from build123d import *

# Parameters (mm, degrees)
BASEFLANGE_W                   = 70
BASEFLANGE_H                   = 531
BASE_FLANGE1_DEPTH             = 2
EDGE_FLANGE1_STRIP_W           = 10
EDGE_FLANGE1_STRIP_H           = 2
EDGE_FLANGE1_STRIP_CUT_DEPTH   = 531
EDGE_FLANGE1_STRIP_2_W         = 10
EDGE_FLANGE1_STRIP_2_H         = 2
EDGE_FLANGE1_STRIP_CUT_2_DEPTH = 531
EDGE_FLANGE1_DEPTH             = 531
EDGE_FLANGE1_BEND_DEPTH        = 531
EDGE_FLANGE2_STRIP_W           = 10
EDGE_FLANGE2_STRIP_H           = 2
EDGE_FLANGE2_STRIP_CUT_DEPTH   = 531
EDGE_FLANGE2_STRIP_2_W         = 10
EDGE_FLANGE2_STRIP_2_H         = 2
EDGE_FLANGE2_STRIP_CUT_2_DEPTH = 531
EDGE_FLANGE2_DEPTH             = 531
EDGE_FLANGE2_BEND_DEPTH        = 531


# Sheet-metal steps are written as plain solids
with BuildPart() as part:
    # BaseFlange → Base-Flange1 (new body)
    with BuildSketch(Plane(origin=(0, 0, 0), x_dir=(1, 0, 0), z_dir=(0, 1, 0))):
        with Locations((0, -265.5)):
            Rectangle(BASEFLANGE_W, BASEFLANGE_H)
    extrude(amount=-BASE_FLANGE1_DEPTH)

    # Edge-Flange1 strip (across the edge) → Edge-Flange1 strip cut (cut)
    with BuildSketch(Plane(origin=(-35, -2, 531), x_dir=(1, 0, 0), z_dir=(0, 0, -1))):
        with Locations((-2, -1)):
            Rectangle(EDGE_FLANGE1_STRIP_W, EDGE_FLANGE1_STRIP_H)
    extrude(amount=EDGE_FLANGE1_STRIP_CUT_DEPTH, mode=Mode.SUBTRACT)

    # Edge-Flange1 strip 2 (across the edge) → Edge-Flange1 strip cut 2 (cut)
    with BuildSketch(Plane(origin=(35, -2, 0), x_dir=(-1, 0, 0), z_dir=(0, 0, 1))):
        with Locations((-2, -1)):
            Rectangle(EDGE_FLANGE1_STRIP_2_W, EDGE_FLANGE1_STRIP_2_H)
    extrude(amount=EDGE_FLANGE1_STRIP_CUT_2_DEPTH, mode=Mode.SUBTRACT)

    # Edge-Flange1 section (across the edge) → Edge-Flange1 (add)
    with BuildSketch(Plane(origin=(-35, -2, 531), x_dir=(1, 0, 0), z_dir=(0, 0, -1))):
        with BuildLine():
            Line((0, 1), (0, 46))
            Line((0, 46), (2, 46))
            Line((2, 46), (2, 1))
            ThreePointArc((2, 1), (2.292893219, 0.292893219), (3, 0))
            Line((3, 0), (3, -2))
            ThreePointArc((3, -2), (0.878679656, -1.121320344), (0, 1))
        make_face()
    extrude(amount=EDGE_FLANGE1_DEPTH)

    # Edge-Flange1 section 2 (across the edge) → Edge-Flange1 bend (add)
    with BuildSketch(Plane(origin=(35, -2, 0), x_dir=(-1, 0, 0), z_dir=(0, 0, 1))):
        with BuildLine():
            Line((0, 1), (0, 46))
            Line((0, 46), (2, 46))
            Line((2, 46), (2, 1))
            ThreePointArc((2, 1), (2.292893219, 0.292893219), (3, 0))
            Line((3, 0), (3, -2))
            ThreePointArc((3, -2), (0.878679656, -1.121320344), (0, 1))
        make_face()
    extrude(amount=EDGE_FLANGE1_BEND_DEPTH)

    # Edge-Flange2 strip (across the edge) → Edge-Flange2 strip cut (cut)
    with BuildSketch(Plane(origin=(-33, -48, 531), x_dir=(0, 1, 0), z_dir=(0, 0, -1))):
        with Locations((-2, -1)):
            Rectangle(EDGE_FLANGE2_STRIP_W, EDGE_FLANGE2_STRIP_H)
    extrude(amount=EDGE_FLANGE2_STRIP_CUT_DEPTH, mode=Mode.SUBTRACT)

    # Edge-Flange2 strip 2 (across the edge) → Edge-Flange2 strip cut 2 (cut)
    with BuildSketch(Plane(origin=(33, -48, 0), x_dir=(0, 1, 0), z_dir=(0, 0, 1))):
        with Locations((-2, -1)):
            Rectangle(EDGE_FLANGE2_STRIP_2_W, EDGE_FLANGE2_STRIP_2_H)
    extrude(amount=EDGE_FLANGE2_STRIP_CUT_2_DEPTH, mode=Mode.SUBTRACT)

    # Edge-Flange2 section (across the edge) → Edge-Flange2 (add)
    with BuildSketch(Plane(origin=(-33, -48, 531), x_dir=(0, 1, 0), z_dir=(0, 0, -1))):
        with BuildLine():
            Line((0, 1), (0, 8))
            Line((0, 8), (2, 8))
            Line((2, 8), (2, 1))
            ThreePointArc((2, 1), (2.292893219, 0.292893219), (3, 0))
            Line((3, 0), (3, -2))
            ThreePointArc((3, -2), (0.878679656, -1.121320344), (0, 1))
        make_face()
    extrude(amount=EDGE_FLANGE2_DEPTH)

    # Edge-Flange2 section 2 (across the edge) → Edge-Flange2 bend (add)
    with BuildSketch(Plane(origin=(33, -48, 0), x_dir=(0, 1, 0), z_dir=(0, 0, 1))):
        with BuildLine():
            Line((0, 1), (0, 8))
            Line((0, 8), (2, 8))
            Line((2, 8), (2, 1))
            ThreePointArc((2, 1), (2.292893219, 0.292893219), (3, 0))
            Line((3, 0), (3, -2))
            ThreePointArc((3, -2), (0.878679656, -1.121320344), (0, 1))
        make_face()
    extrude(amount=EDGE_FLANGE2_BEND_DEPTH)


solid = part.part
Part model, mm, in its own coordinate system. A direction names the side the tool comes from. Coordinates: 2 decimals unless noted, no trailing zeros. Order: outer loops, then holes, each group sorted by start corner. A loop starts at its lowest first (then second) coordinate and runs counter-clockwise, first axis right, second up.
(1) Pull direction X, two halves, no side cores. Call faces 3 (the face through (0, -1, 531)), 4 (the face through (-35, -24, 269)), 5 (the face through (33, -24, 262)): pulls with the +X half, pulls with the -X half, needs draft (parallel to the pull), parting line crosses it, or undercut.
Check sheet entries:
face 3: needs draft
face 4: pulls with the -X half
face 5: undercut
(2) Tool access for faces 1 (the face through (-33, -24, 269)), 2 (the face through (0, -1, 0)): list every direction of +Z, -Z, +X, -X, +Y, -Y with a clear straight run to the whole face (end or side of a thin tool).
Check sheet entries:
face 1: +Z, -Z
face 2: -Z, +X, -X, +Y, -Y
(3) Probe L1, parallel to X at y = -14, z = 190.5; L2, parallel to Y at x = 30, z = 183.5; L3, parallel to Y at x = -22, z = 88. List the from-to ranges inside material, lowest first.
Check sheet entries:
L1: x = -35 to -33, 33 to 35
L2: y = -48 to -46, -2 to 0
L3: y = -2 to 0
(4) Slice it at C-C, the plane x = 3. Write the cut outline in (y, z), and give its area (3 significant figures).
Check sheet entries:
outline: (-2, 0) - (0, 0) - (0, 531) - (-2, 531) - close
area: 1,060 mm2
(5) Slice it at B-B, the plane z = 35. Write the cut outline in (x, y).
Check sheet entries:
outline: (-35, -45) arc R3 ccw to (-32, -48) - (-25, -48) - (-25, -46) - (-32, -46) arc R1 cw to (-33, -45) - (-33, -3) arc R1 cw to (-32, -2) - (32, -2) arc R1 cw to (33, -3) - (33, -45) arc R1 cw to (32, -46) - (25, -46) - (25, -48) - (32, -48) arc R3 ccw to (35, -45) - (35, -3) arc R3 ccw to (32, 0) - (-32, 0) arc R3 ccw to (-35, -3) - close
(6) Slice it at A-A, the plane y = -12.5. Write the cut outline in (x, z).
Check sheet entries:
outline: (-35, 0) - (-33, 0) - (-33, 531) - (-35, 531) - close; (33, 0) - (35, 0) - (35, 531) - (33, 531) - close
(7) Pin check, flat tips, straight feed: pin 1 Ø0.6 at (y, z) = (-47, 185.5) entering from +X; pin 2 Ø2 at (x, z) = (4.5, 55) entering from -Y; pin 3 Ø1.6 at (y, z) = (-47.5, 221) entering from -X. Stop position of each tip, or through.
Check sheet entries:
pin 1: stops at x = 34.47
pin 2: stops at y = -2
pin 3: stops at x = -34.47
